Source: CAD feature listing. Evaluate the final solid. Frame: model axes, mm. A direction names the side the tool comes from. Round coordinates to 2 decimals unless told otherwise and drop trailing zeros. Write each loop counter-clockwise with the first axis right and the second up, starting at its lowest first coordinate (ties: lowest second). Pieces come first, ordered by that corner, then holes.
from build123d import *

# Parameters (mm, degrees)
SKETCH1_W           = 200
SKETCH1_H           = 50
BOSS_EXTRUDE1_DEPTH = 5
SKETCH2_W           = 50
SKETCH2_H           = 60
BOSS_EXTRUDE2_DEPTH = 10
CUT_EXTRUDE1_START  = -201
CUT_EXTRUDE1_DEPTH  = 202
FILLET1_R           = 2


with BuildPart() as part:
    # Sketch1 → Boss-Extrude1 (new body)
    with BuildSketch(Plane(origin=(0, 0, 0), x_dir=(1, 0, 0), z_dir=(0, 1, 0))):
        Rectangle(SKETCH1_W, SKETCH1_H)
    extrude(amount=BOSS_EXTRUDE1_DEPTH)

    # Sketch2 → Boss-Extrude2 (add)
    with BuildSketch(Plane.ZY.offset(100)):
        with Locations((0, 35)):
            Rectangle(SKETCH2_W, SKETCH2_H)
    boss_extrude2 = extrude(amount=-BOSS_EXTRUDE2_DEPTH)

    # Sketch3 → Cut-Extrude1 (cut)
    with BuildSketch(Plane.ZY.offset(100).offset(CUT_EXTRUDE1_START)):
        Polygon((25, 39.80474613), (6.89100161, 55), (-2.5, 55), (-2.5, 46.935822228), (2.5, 46.935822228), (5.071150439, 50), (25, 33.277709683), align=None)
    cut_extrude1 = extrude(amount=CUT_EXTRUDE1_DEPTH, mode=Mode.SUBTRACT)

    # Mirror1: Boss-Extrude2, Cut-Extrude1 across plane
    add(boss_extrude2.mirror(Plane(origin=(0, 0, 0), x_dir=(0, 0, 1), z_dir=(1, 0, 0))))
    add(cut_extrude1.mirror(Plane(origin=(0, 0, 0), x_dir=(0, 0, 1), z_dir=(1, 0, 0))), mode=Mode.SUBTRACT)

    # Fillet1
    fillet1_edges = [part.edges().sort_by_distance(p)[0] for p in [
        (-90, 5, 0),
        (-90, 65, 0),
        (-100, 65, 0),
        (100, 0, 0),
        (100, 65, 0),
        (-100, 0, 0),
        (90, 5, 0),
        (90, 65, 0),
    ]]
    fillet(fillet1_edges, radius=FILLET1_R)


solid = part.part
1) Reachability of faces 1 (the face through (90, 35, 0)), 2 (the face through (8, 4, 25)), 3 (the face through (-95, 51, -2.5)) from +Z, -Z, +X, -X, +Y, -Y: full face, straight path, thin tool, end or side. Return the list, or none.
Taken from the geometry:
face 1: +Z, -Z, +Y
face 2: +Z, +X, -X, +Y, -Y
face 3: +X, -X
2) Section query B-B on y = 43.5. Return the cut outline in (x, z).
Taken from the geometry:
outline: (-100, -25) - (-90, -25) - (-90, 12.82) - (-100, 12.82) - close; (-100, 20.6) - (-90, 20.6) - (-90, 25) - (-100, 25) - close; (90, -25) - (100, -25) - (100, 12.82) - (90, 12.82) - close; (90, 20.6) - (100, 20.6) - (100, 25) - (90, 25) - close
3) Pull-direction query (Y, two-part tool) for faces 4 (the face through (100, 33, 0)), 5 (the face through (-1, 5, 0)), 6 (the face through (95, 51, -2.5)); classes: released by +Y, released by -Y, zero draft, split by the parting line, or undercut.
Taken from the geometry:
face 4: zero draft
face 5: released by +Y
face 6: undercut
4) Section query C-C on z = -16.5. Return the cut outline in (x, y), then the cut area to 3 significant figures.
Taken from the geometry:
outline: (-100, 2) arc R2 ccw to (-98, 0) - (98, 0) arc R2 ccw to (100, 2) - (100, 63) arc R2 ccw to (98, 65) - (92, 65) arc R2 ccw to (90, 63) - (90, 7) arc R2 cw to (88, 5) - (-88, 5) arc R2 cw to (-90, 7) - (-90, 63) arc R2 ccw to (-92, 65) - (-98, 65) arc R2 ccw to (-100, 63) - close
area: 2,200 mm2
5) Section query D-D on z = 17.5. Return the cut outline in (x, y), then the cut area to 3 significant figures.
Taken from the geometry:
outline: (-100, 2) arc R2 ccw to (-98, 0) - (98, 0) arc R2 ccw to (100, 2) - (100, 39.57) - (90, 39.57) - (90, 7) arc R2 cw to (88, 5) - (-88, 5) arc R2 cw to (-90, 7) - (-90, 39.57) - (-100, 39.57) - close; (-100, 46.1) - (-90, 46.1) - (-90, 63) arc R2 ccw to (-92, 65) - (-98, 65) arc R2 ccw to (-100, 63) - close; (90, 46.1) - (100, 46.1) - (100, 63) arc R2 ccw to (98, 65) - (92, 65) arc R2 ccw to (90, 63) - close
area: 2,070 mm2
6) Section query A-A on y = 24. Return the cut outline in (x, z), then the cut area to 3 significant figures.
Taken from the geometry:
outline: (-100, -25) - (-90, -25) - (-90, 25) - (-100, 25) - close; (90, -25) - (100, -25) - (100, 25) - (90, 25) - close
area: 1,000 mm2
7) Material intervals for line 1 (X direction, y = 22.5, z = -7.5); line 2 (Y direction, x = 40, z = 1.5), sorted ascending.
Taken from the geometry:
line 1: x = -100 to -90, 90 to 100
line 2: y = 0 to 5
8) Contact query for flat-ended pins moving along their axis: P1, Ø2, axis at x = 9, z = 10, coming from the +Y side; P2, Ø6, axis at x = -63.5, y = 8.5, coming from the +Z side. Output: stop coordinate, or through.
Taken from the geometry:
P1: stops at y = 5
P2: passes through
